from build123d import *

# Parameters (mm, degrees)
F0_W     = 102
F0_H     = 40
F1_DEPTH = 3
F2_W     = 3
F2_H     = 5
F3_DEPTH = 3
F4_W     = 5
F4_H     = 3
F5_DEPTH = 3
F6_W     = 3
F6_H     = 5
F7_DEPTH = 25


with BuildPart() as f1:
    # F0 (on Front) → F1 (new body)
    with BuildSketch(Plane.XZ):
        Rectangle(F0_W, F0_H)
    extrude(amount=F1_DEPTH)

    # F2 (on face) → F3 (join)
    with BuildSketch(Plane.XZ.offset(3)):
        with Locations((-52.5, -17.5)):
            Rectangle(F2_W, F2_H)
        with Locations((-52.5, -7.5)):
            Rectangle(F2_W, F2_H)
        with Locations((-52.5, 2.5)):
            Rectangle(F2_W, F2_H)
        with Locations((-52.5, 12.5)):
            Rectangle(F2_W, F2_H)
        with Locations((52.5, -7.5)):
            Rectangle(F2_W, F2_H)
        with Locations((52.5, -17.5)):
            Rectangle(F2_W, F2_H)
        with Locations((52.5, 12.5)):
            Rectangle(F2_W, F2_H)
        with Locations((52.5, 2.5)):
            Rectangle(F2_W, F2_H)
    extrude(amount=-F3_DEPTH)

    # F4 (on face) → F5 (join)
    with BuildSketch(Plane(origin=(0, 0, 0), x_dir=(-1, 0, 0), z_dir=(0, 1, 0))):
        with Locations((0, 21.5)):
            Rectangle(F4_W, F4_H)
        with Locations((10, 21.5)):
            Rectangle(F4_W, F4_H)
        with Locations((20, 21.5)):
            Rectangle(F4_W, F4_H)
        with Locations((30, 21.5)):
            Rectangle(F4_W, F4_H)
        with Locations((40, 21.5)):
            Rectangle(F4_W, F4_H)
        Polygon((52.5, 23), (47.5, 23), (47.5, 20), (52.5, 20), (54, 20), (54, 23), align=None)
        Polygon((-52.5, 20), (-47.5, 20), (-47.5, 23), (-52.5, 23), (-54, 23), (-54, 20), align=None)
        with Locations((-20, 21.5)):
            Rectangle(F4_W, F4_H)
        with Locations((-10, 21.5)):
            Rectangle(F4_W, F4_H)
        with Locations((-30, 21.5)):
            Rectangle(F4_W, F4_H)
        with Locations((-40, 21.5)):
            Rectangle(F4_W, F4_H)
    extrude(amount=-F5_DEPTH)

    # F6 (on face) → F7 (cut)
    with BuildSketch(Plane.XZ.offset(3)):
        with Locations((-32, -12.5)):
            Rectangle(F6_W, F6_H)
        with Locations((-32, -2.5)):
            Rectangle(F6_W, F6_H)
        with Locations((-38, -12.5)):
            Rectangle(F6_W, F6_H)
        with Locations((-38, -2.5)):
            Rectangle(F6_W, F6_H)
        with Locations((32, -12.5)):
            Rectangle(F6_W, F6_H)
        with Locations((32, -2.5)):
            Rectangle(F6_W, F6_H)
        with Locations((38, -12.5)):
            Rectangle(F6_W, F6_H)
        with Locations((38, -2.5)):
            Rectangle(F6_W, F6_H)
    extrude(amount=-F7_DEPTH, mode=Mode.SUBTRACT)


solid = f1.part
Geometry: final body of the model. Coordinates: model frame, mm. A direction names the side the tool comes from. Give positions to 0.01 mm unless a question says otherwise; leave off trailing zeros. Order: outer loops, then holes, each group sorted by start corner. A loop starts at its lowest first (then second) coordinate and runs counter-clockwise, first axis right, second up. Notation, with made-up numbers: (18.5, 73.5) - (50.5, 73.5) arc R15 ccw to (50.5, 84.5) - close; hole circle Ø6 at (-14.5, 73.25). An arc over 180 degrees is marked (long way). Use CSV: the item, a comma, the result in double quotes.
1. Material intervals for line 1 along X through (y, z) = (-1.75, -11); line 2 along Z through (x, y) = (-15, -0.4); line 3 along X through (y, z) = (-1.65, 18), sorted ascending. Write a range as from..to.
Answers below:
line 1,"-51..-39.5, -36.5..-33.5, -30.5..30.5, 33.5..36.5, 39.5..51"
line 2,"-20..20"
line 3,"-51..51"
2. Access query for faces 5 (the face through (-51, -1, 7)), 6 (the face through (-38, -2, 0)), 7 (the face through (-32.5, -1, 21)). Directions: +Z, -Z, +X, -X, +Y, -Y. A direction counts if a zero-diameter tool reaches every point of the face in a straight line with its end or side. Return the directions, or none.
Answers below:
face 5,"-X, +Y, -Y"
face 6,"+Y, -Y"
face 7,"+Z, +Y, -Y"
3. Section query A-A (x = -38.5). Output: boundary loops of the cut face in (y, z), plus the area to 3 significant figures.
Answers below:
outline,"(-3, -20) - (0, -20) - (0, -15) - (-3, -15) - close; (-3, -10) - (0, -10) - (0, -5) - (-3, -5) - close; (-3, 0) - (0, 0) - (0, 23) - (-3, 23) - close"
area,"99.0 mm2"
4. Section query C-C (y = -0.7). Give the number of separate pieces and of enclosed holes in the cut face, plus the area to 3 significant figures.
Answers below:
separate pieces,"1"
enclosed holes,"8"
area,"4,250 mm2"
5. Mould query, pull axis Z, two halves, no side actions, for faces 1 (the face through (38, -2, -5)), 2 (the face through (-53, -2, 15)), 3 (the face through (-15, -1, 20)), 4 (the face through (-12.5, -1, 21)). Classes: +Z half, -Z half, draft (parallel to the pull), parting line (faces both ways), or undercut.
Answers below:
face 1,"undercut"
face 2,"undercut"
face 3,"+Z half"
face 4,"draft"
6. Section query B-B (z = -4). Output: boundary loops of the cut face in (x, y), plus the area to 3 significant figures.
Answers below:
outline,"(-51, -3) - (-39.5, -3) - (-39.5, 0) - (-51, 0) - close; (-36.5, -3) - (-33.5, -3) - (-33.5, 0) - (-36.5, 0) - close; (-30.5, -3) - (30.5, -3) - (30.5, 0) - (-30.5, 0) - close; (33.5, -3) - (36.5, -3) - (36.5, 0) - (33.5, 0) - close; (39.5, -3) - (51, -3) - (51, 0) - (39.5, 0) - close"
area,"270 mm2"
7. Contact query for flat-ended pins moving along their axis: pin 1 (0.9 mm diameter, centred on y = -2, z = 16.5, fed in from -X); pin 2 (0.9 mm diameter, centred on y = -1.5, z = -3.5, fed in from +X). Output: stop coordinate, or through.
Answers below:
pin 1,"x = -51"
pin 2,"x = 51"
